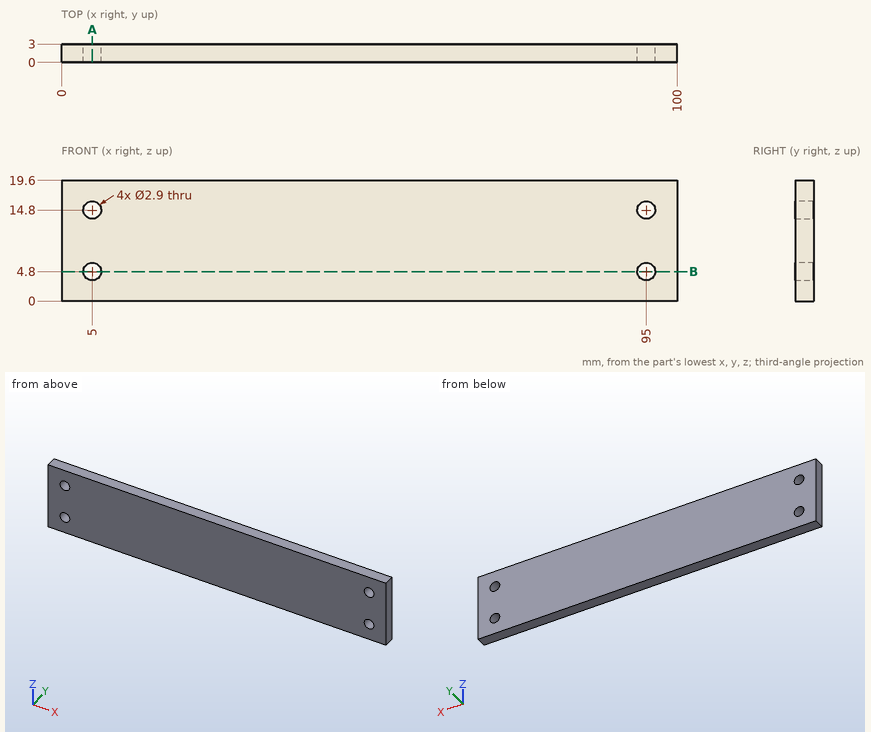
Input: dimensioned drawing with shaded views. Units: mm. Origin: part minimum x, y, z. Coordinates: 2 decimals unless noted, no trailing zeros. Order: outer loops, then holes, each group sorted by start corner. A loop starts at its lowest first (then second) coordinate and runs counter-clockwise, first axis right, second up.
Item 1: Section query B-B (z = 4.8). Output: boundary loops of the cut face in (x, y).
Answer:
outline: (0, 0) - (3.55, 0) - (3.55, 3) - (0, 3) - close; (6.45, 0) - (93.55, 0) - (93.55, 3) - (6.45, 3) - close; (96.45, 0) - (100, 0) - (100, 3) - (96.45, 3) - close
Item 2: Section query A-A (x = 5). Output: boundary loops of the cut face in (y, z).
Answer:
outline: (0, 0) - (3, 0) - (3, 3.35) - (0, 3.35) - close; (0, 6.25) - (3, 6.25) - (3, 13.35) - (0, 13.35) - close; (0, 16.25) - (3, 16.25) - (3, 19.6) - (0, 19.6) - close
Item 3: Contact query for a flat-ended pin moving along its axis: P1, Ø1.7, axis at x = 5, z = 14.8, coming from the -Y side. Output: stop coordinate, or through.
Answer:
P1: passes through
Item 4: Material intervals for line 1 along Z through (x, y) = (5, 0.9); line 2 along X through (y, z) = (2.2, 14.8); line 3 along Z through (x, y) = (96, 0.65), sorted ascending.
Answer:
line 1: z = 0 to 3.35, 6.25 to 13.35, 16.25 to 19.6
line 2: x = 0 to 3.55, 6.45 to 93.55, 96.45 to 100
line 3: z = 0 to 3.75, 5.85 to 13.75, 15.85 to 19.6
